from build123d import *

# Parameters (mm, degrees)
SKICA2_W                 = 3
SKICA2_H                 = 48.4
SKICA2_H_2               = 6
P_IDAT_VYSUNUT_M1_DEPTH  = 2.5
SKICA2_3_W               = 3
SKICA2_3_H               = 6
P_IDAT_VYSUNUT_M2_DEPTH  = 8.8275
SKICA3_R                 = 1.35
ODEBRAT_VYSUNUT_M1_DEPTH = 8.8275


with BuildPart() as part:
    # Skica2 → P_idat vysunut_m1 (new body)
    with BuildSketch(Plane.XY):
        with Locations((-1.5, -30.2)):
            Rectangle(SKICA2_W, SKICA2_H)
        with Locations((-1.5, -3)):
            Rectangle(SKICA2_W, SKICA2_H_2)
        with Locations((-1.5, -57.4)):
            Rectangle(SKICA2_W, SKICA2_H_2)
    extrude(amount=P_IDAT_VYSUNUT_M1_DEPTH)

    # Skica2_3 → P_idat vysunut_m2 (add)
    with BuildSketch(Plane.XY):
        with Locations((-1.5, -3)):
            Rectangle(SKICA2_3_W, SKICA2_3_H)
        with Locations((-1.5, -57.4)):
            Rectangle(SKICA2_3_W, SKICA2_3_H)
    extrude(amount=P_IDAT_VYSUNUT_M2_DEPTH)

    # Skica3 → Odebrat vysunut_m1 (cut)
    with BuildSketch(Plane.ZY.offset(3)):
        with Locations((5.66375, -3)):
            Circle(SKICA3_R)
        with Locations((5.66375, -57.4)):
            Circle(SKICA3_R)
    extrude(amount=-ODEBRAT_VYSUNUT_M1_DEPTH, mode=Mode.SUBTRACT)


solid = part.part
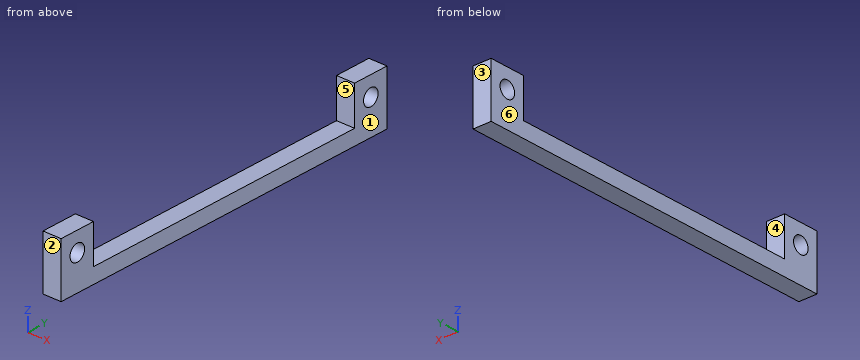
The listing builds one solid part. Answer for the finished solid, in the listing's coordinates (mm). Face numbers are marked on the shaded views. A direction names the side the tool comes from. Round coordinates to 2 decimals unless told otherwise and drop trailing zeros. Order: outer loops, then holes, each group sorted by start corner. A loop starts at its lowest first (then second) coordinate and runs counter-clockwise, first axis right, second up. Notation, with made-up numbers: (22.25, 83.25) -> (63.25, 83.25) arc R22 ccw to (63.25, 111.25) -> close; hole circle Ø1 at (37, -5.75). An arc over 180 degrees is marked (long way). Put each result on its own line as item: value.
Q1. Consider line 1 along Y through (x, z) = (-1.95, 5.75); line 2 along Y through (x, z) = (-2.4, 3.75); line 3 along Y through (x, z) = (-1.6, 4.5). Determine where each line is inside the solid, lowest interval first.
Results list:
line 1: -60.4 to -58.75, -56.05 to -54.4, -6 to -4.35, -1.65 to 0
line 2: -60.4 to -54.4, -6 to 0
line 3: -60.4 to -58.08, -56.72 to -54.4, -6 to -3.68, -2.32 to 0
Q2. Section B-B, the plane x = -2.5 is taken. Write down the section's boundary in (y, z), and give its area (3 significant figures).
Results list:
outline: (-60.4, 0) -> (0, 0) -> (0, 8.83) -> (-6, 8.83) -> (-6, 2.5) -> (-54.4, 2.5) -> (-54.4, 8.83) -> (-60.4, 8.83) -> close; hole circle Ø2.7 at (-57.4, 5.66); hole circle Ø2.7 at (-3, 5.66)
area: 215 mm^2
Q3. This flat-tipped pin is pushed along its axis until it touches: P1, Ø5, axis at y = -27.5, z = 5.5, coming from the +X side. Where does it stop, or does it pass through?
Results list:
P1: through
Q4. Section D-D, the plane y = -10 is taken. Write down the section's boundary in (x, z).
Results list:
outline: (-3, 0) -> (0, 0) -> (0, 2.5) -> (-3, 2.5) -> close
Q5. Section A-A, the plane z = 7.75 is taken. Write down the section's boundary in (x, y).
Results list:
outline: (-3, -60.4) -> (0, -60.4) -> (0, -54.4) -> (-3, -54.4) -> close; (-3, -6) -> (0, -6) -> (0, 0) -> (-3, 0) -> close
Q6. Section C-C, the plane y = -57.4 is taken. Write down the section's boundary in (x, z).
Results list:
outline: (-3, 0) -> (0, 0) -> (0, 4.31) -> (-3, 4.31) -> close; (-3, 7.01) -> (0, 7.01) -> (0, 8.83) -> (-3, 8.83) -> close
Q7. Determine the mould class of the marked faces 1, 2, 3 and 4 for opening direction Y: pulls with the +Y half, pulls with the -Y half, needs draft (parallel to the pull), parting line crosses it, or undercut.
Results list:
face 1: needs draft
face 2: pulls with the -Y half
face 3: pulls with the +Y half
face 4: undercut
Q8. Which of the six approach directions +Z, -Z, +X, -X, +Y, -Y give full straight-line access (tool end or side, diameter ignored) to the marked faces 5 and 6?
Results list:
face 5: +Z, +X, -X
face 6: +Z, -Z, -X, +Y, -Y
